Check sheet for the modelled part. Datum: model origin and axes. Units: mm. Face numbers are marked on the shaded views. A direction names the side the tool comes from. Round coordinates to 2 decimals unless told otherwise and drop trailing zeros. Order: outer loops, then holes, each group sorted by start corner. A loop starts at its lowest first (then second) coordinate and runs counter-clockwise, first axis right, second up.
Q1. Mould release check, pull along X, two halves, no side actions. Record for the marked faces 3, 4, 5 and 6: +X half, -X half, draft (parallel to the pull), parting line (faces both ways), or undercut.
Q2. Set-up check for the marked faces 1 and 2: record each of +Z, -Z, +X, -X, +Y, -Y from which the full face is reachable in a straight line by a thin tool's end or side.
Q3. Depth check by flat-ended pin: P1, Ø9, axis at x = -63, y = -66, coming from the +Z side. Enter the tip coordinate at first touch or a pass-through.
Q4. Cross-section at A-A on y = 0. Record the cut outline in (x, z), then the cut area to 3 significant figures.
Q5. Scan lines: probe 1 along Y at (x, z) = (0, 66); probe 2 along Y at (x, z) = (-55, 64.5); probe 3 along Z at (x, y) = (-36, -17). Record each from-to range of solid material in increasing order.
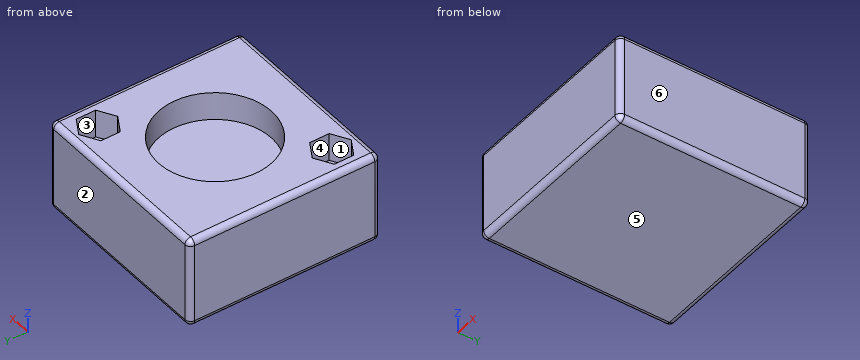
from build123d import *

# Parameters (mm, degrees)
F0_W     = 170
F0_H     = 170
F1_DEPTH = 80
F2_R     = 50
F3_DEPTH = 25
F4_R     = 5
F5_R     = 5


with BuildPart() as f1:
    # F0 (on Top) → F1 (new body)
    with BuildSketch(Plane.XY):
        Rectangle(F0_W, F0_H)
    extrude(amount=F1_DEPTH)

    # F2 (on face) → F3 (cut)
    with BuildSketch(Plane.XY.offset(80)):
        Circle(F2_R)
        Polygon((-75, -51.339746), (-75, -68.660254), (-60, -77.320508), (-45, -68.660254), (-45, -51.339746), (-60, -42.679492), align=None)
        Polygon((75, 51.339746), (75, 68.660254), (60, 77.320508), (45, 68.660254), (45, 51.339746), (60, 42.679492), align=None)
    extrude(amount=-F3_DEPTH, mode=Mode.SUBTRACT)

    # F4
    f4_edges = [f1.edges().sort_by_distance(p)[0] for p in [
        (85, -85, 40),
        (85, 85, 40),
        (-85, 85, 40),
        (-85, -85, 40),
    ]]
    fillet(f4_edges, radius=F4_R)

    # F5
    f5_edges = [f1.edges().sort_by_distance(p)[0] for p in [
        (-85, 0, 80),
        (85, 0, 0),
    ]]
    fillet(f5_edges, radius=F5_R)


solid = f1.part
Results found:
1. face 3: undercut
1. face 4: undercut
1. face 5: draft
1. face 6: +X half
2. face 1: +Z
2. face 2: +Z, -Z, +X, -X, +Y
3. P1: stops at z = 55
4. outline: (-85, 5) arc R5 ccw to (-80, 0) - (80, 0) arc R5 ccw to (85, 5) - (85, 75) arc R5 ccw to (80, 80) - (50, 80) - (50, 55) - (-50, 55) - (-50, 80) - (-80, 80) arc R5 ccw to (-85, 75) - close
4. area: 11,100 mm2
5. probe 1: y = -85 to -50, 50 to 85
5. probe 2: y = -85 to -74.43, -45.57 to 85
5. probe 3: z = 0 to 55
